For this review, take the finished solid that the model builds, in its own axes (mm). Face numbers are marked on the shaded views. A direction names the side the tool comes from. Give positions to 0.01 mm unless a question says otherwise; leave off trailing zeros. Order: outer loops, then holes, each group sorted by start corner. A loop starts at its lowest first (then second) coordinate and runs counter-clockwise, first axis right, second up.
Item 1: Machinability: for the marked faces 1, 2 and 3, which of the approach directions +Z, -Z, +X, -X, +Y, -Y give a long, thin tool a straight path to every point of the face, cutting with its end or side? Answer none if there is none.
Item 2: Consider section A-A (z = -18). Give the boundary of the cut face in (x, y), plus the area to 3 significant figures.
Item 3: For P1, Ø1.5, axis at x = 2, y = 0.5, coming from the -Z side, flat-tipped, find the tip position at first contact; note if it passes through.
Item 4: For probe 1 along Z at (x, y) = (-17, 1.7); probe 2 along X at (y, z) = (2.05, -10); probe 3 along X at (y, z) = (1.3, -15), list the stretches that pass through material, from the lowest coordinate up.
Item 5: The part is to be moulded in two halves that separate along X. For the marked faces 4, 5 and 6, say which applies: released by +X, released by -X, zero draft, split by the parting line, or undercut.
Item 6: Consider section C-C (z = 12.5). Give the boundary of the cut face in (x, y), plus the area to 3 significant figures.
Item 7: Consider section B-B (z = 0). Give the boundary of the cut face in (x, y), plus the area to 3 significant figures.
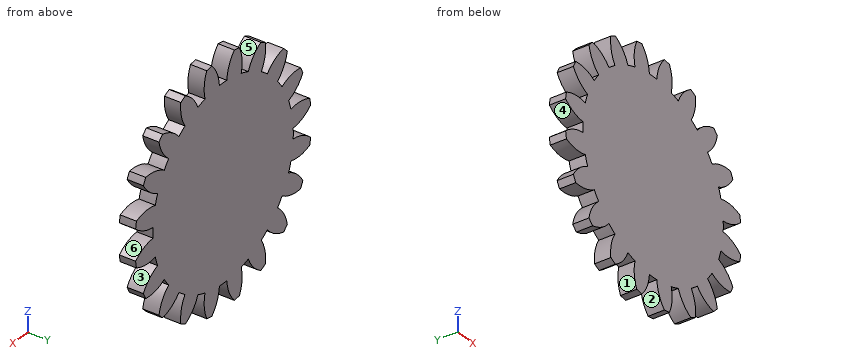
```python
from build123d import *

# Parameters (mm, degrees)
CROQUIS1_R              = 22
SALIENTE_EXTRUIR1_DEPTH = 3
CORTAR_EXTRUIR1_DEPTH   = 3
MATRIZC1_COUNT          = 20


with BuildPart() as part:
    # Croquis1 → Saliente-Extruir1 (new body)
    with BuildSketch(Plane(origin=(0, 0, 0), x_dir=(1, 0, 0), z_dir=(0, 1, 0))):
        with Locations(Location((0, 0, 0), (0, 0, 270))):  # turned: the seam where the file's is
            Circle(CROQUIS1_R)
    extrude(amount=SALIENTE_EXTRUIR1_DEPTH)

    # Croquis2 → Cortar-Extruir1 (cut)
    with BuildSketch(Plane(origin=(0, 3, 0), x_dir=(1, 0, 0), z_dir=(0, 1, 0))):
        with BuildLine():
            ThreePointArc((0.928527245, 17.475349414), (1.485995248, 19.810616222), (2.797926902, 21.821356627))
            ThreePointArc((2.797926902, 21.821356627), (0, 22), (-2.797926902, 21.821356627))
            ThreePointArc((-2.797926902, 21.821356627), (-1.485995248, 19.810616222), (-0.928527245, 17.475349414))
            ThreePointArc((-0.928527245, 17.475349414), (0, 17.5), (0.928527245, 17.475349414))
        make_face()
    cortar_extruir1 = extrude(amount=-CORTAR_EXTRUIR1_DEPTH, mode=Mode.SUBTRACT)

    # MatrizC1: Cortar-Extruir1 ×20 about axis
    matrizc1_axis = Axis((0, 0, 0), (0, 1, 0))
    for i in range(1, MATRIZC1_COUNT):
        add(cortar_extruir1.rotate(matrizc1_axis, i * 360 / MATRIZC1_COUNT), mode=Mode.SUBTRACT)


solid = part.part
```
Resolved:
1. face 1: +Y, -Y
1. face 2: -Z, +Y, -Y
1. face 3: +X, +Y, -Y
2. outline: (-10.6, 0) - (-7.22, 0) - (-7.22, 3) - (-10.6, 3) - close; (-4.71, 0) - (-0.98, 0) - (-0.98, 3) - (-4.71, 3) - close; (0.98, 0) - (4.71, 0) - (4.71, 3) - (0.98, 3) - close; (7.22, 0) - (10.6, 0) - (10.6, 3) - (7.22, 3) - close
2. area: 42.6 mm2
3. P1: stops at z = -21.77
4. probe 1: z = -10.46 to -6.59, -4.54 to 4.54, 6.59 to 10.46
4. probe 2: x = -19.6 to -15.57, -14.36 to 14.36, 15.57 to 19.6
4. probe 3: x = -15.99 to -12.6, -9.71 to 9.71, 12.6 to 15.99
5. face 4: released by -X
5. face 5: undercut
5. face 6: released by +X
6. outline: (-14.93, 0) - (14.93, 0) - (14.93, 3) - (-14.93, 3) - close
6. area: 89.6 mm2
7. outline: (-17.5, 0) - (17.5, 0) - (17.5, 3) - (-17.5, 3) - close
7. area: 105 mm2
